Can you work these out from the drawing? Everything is in mm from the part's minimum corner. Round coordinates to 2 decimals unless told otherwise and drop trailing zeros. Loops run counter-clockwise (first coordinate to the right, second up) from the corner with the lowest first, then second, coordinate; pieces in that order, holes last. Notation, with made-up numbers: (-23, 84.25) -> (0, 84.25) arc R20 ccw to (0, 116.25) -> close; hole circle Ø1 at (41.25, 35). An arc over 180 degrees is marked (long way). One line per item, written item: value.
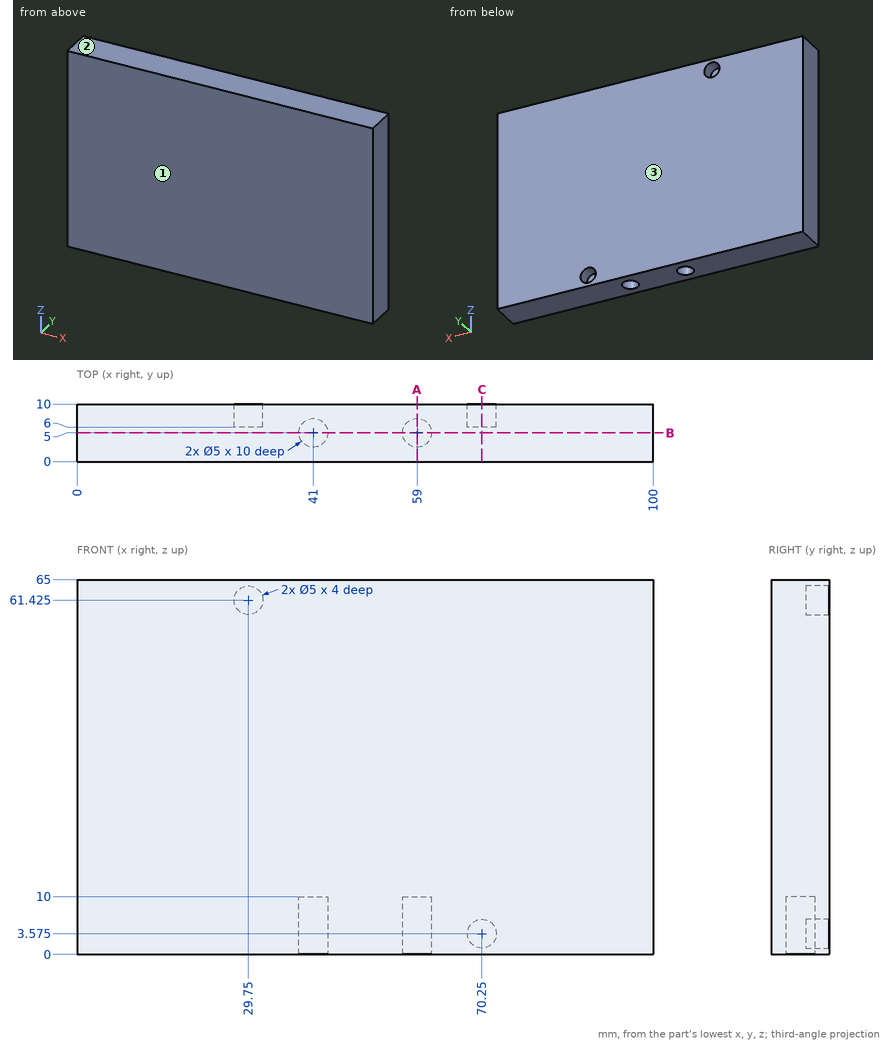
Item 1: If we section it at A-A on x = 59: List the corners of the cut face in (y, z) for me, plus the area to 3 significant figures.
Output:
outline: (0, 0) -> (2.5, 0) -> (2.5, 10) -> (7.5, 10) -> (7.5, 0) -> (10, 0) -> (10, 65) -> (0, 65) -> close
area: 600 mm²
Item 2: If we section it at C-C on x = 70.25: List the corners of the cut face in (y, z) for me (3 decimals).
Output:
outline: (0, 0) -> (10, 0) -> (10, 1.075) -> (6, 1.075) -> (6, 6.075) -> (10, 6.075) -> (10, 65) -> (0, 65) -> close
Item 3: If we mould it in two halves opening along Y, with no side actions, what happens to the marked faces 1, 2 and 3? For each: released by +Y, released by -Y, zero draft, split by the parting line, or undercut.
Output:
face 1: released by -Y
face 2: zero draft
face 3: released by +Y
Item 4: I need wall thicknesses on line 1 (Y direction, x = 41, z = 7.25); line 2 (Z direction, x = 58, y = 5.25). Which ranges of each line are inside material? Lowest first, please. Write a range as from..to.
Output:
line 1: y = 0..2.5, 7.5..10
line 2: z = 10..65
Item 5: If we section it at B-B on y = 5: List the corners of the cut face in (x, z) for me.
Output:
outline: (0, 0) -> (38.5, 0) -> (38.5, 10) -> (43.5, 10) -> (43.5, 0) -> (56.5, 0) -> (56.5, 10) -> (61.5, 10) -> (61.5, 0) -> (100, 0) -> (100, 65) -> (0, 65) -> close
Item 6: Will these pins go through, and if not, where does the flat tip stop? pin 1 Ø4.5 at (x, z) = (29.75, 61.425) entering from +Y; pin 2 Ø2.5 at (x, y) = (42, 4.5) entering from -Z.
Output:
pin 1: stops at y = 6
pin 2: stops at z = 10
